Answer from the drawing. Dimensions are ordinates in mm from the lowest x, y and z of the part. Round coordinates to 2 decimals unless told otherwise and drop trailing zeros. Order: outer loops, then holes, each group sorted by start corner. A loop starts at its lowest first (then second) coordinate and runs counter-clockwise, first axis right, second up. Notation, with made-up numbers: (-22.5, 61) -> (10.5, 61) arc R6 cw to (10.5, 65) -> close; hole circle Ø5 at (-20.75, 27). An arc over 180 degrees is marked (long way). Use a Markdown table: item, result. Add a question column.
1. Section A-A, the plane x = 41 is taken. Give the vertices of the cut face in (y, z), then the cut area to 3 significant figures.
2. Section B-B, the plane z = 41 is taken. Give the vertices of the cut face in (x, y).
3. Section C-C, the plane y = 37 is taken. Give the vertices of the cut face in (x, z), then the cut area to 3 significant figures.
4. The mould has two halves that part along X. Classify the marked faces 1 and 2: +X half, -X half, draft (parallel to the pull), parting line (faces both ways), or undercut.
5. Consider L1, parallel to Z at x = 41, y = 47.5; L2, parallel to X at y = 42, z = 40; L3, parallel to Z at x = 45, y = 32.5. Determine where each line is inside the solid, lowest interval first. Write a range as [from, to].
6. Section D-D, the plane y = 20.5 is taken. Give the vertices of the cut face in (x, z).
7. Given pin 1 (2 mm diameter, centred on y = 12.5, z = 10.5, fed in from +X); pin 2 (1.1 mm diameter, centred on x = 79, y = 43, fed in from +Z); pin 3 (4 mm diameter, centred on x = 35, y = 57.5, fed in from +Z), each flat-ended and moving along its own axis, determine where each tip first touches the part or whether it passes through.
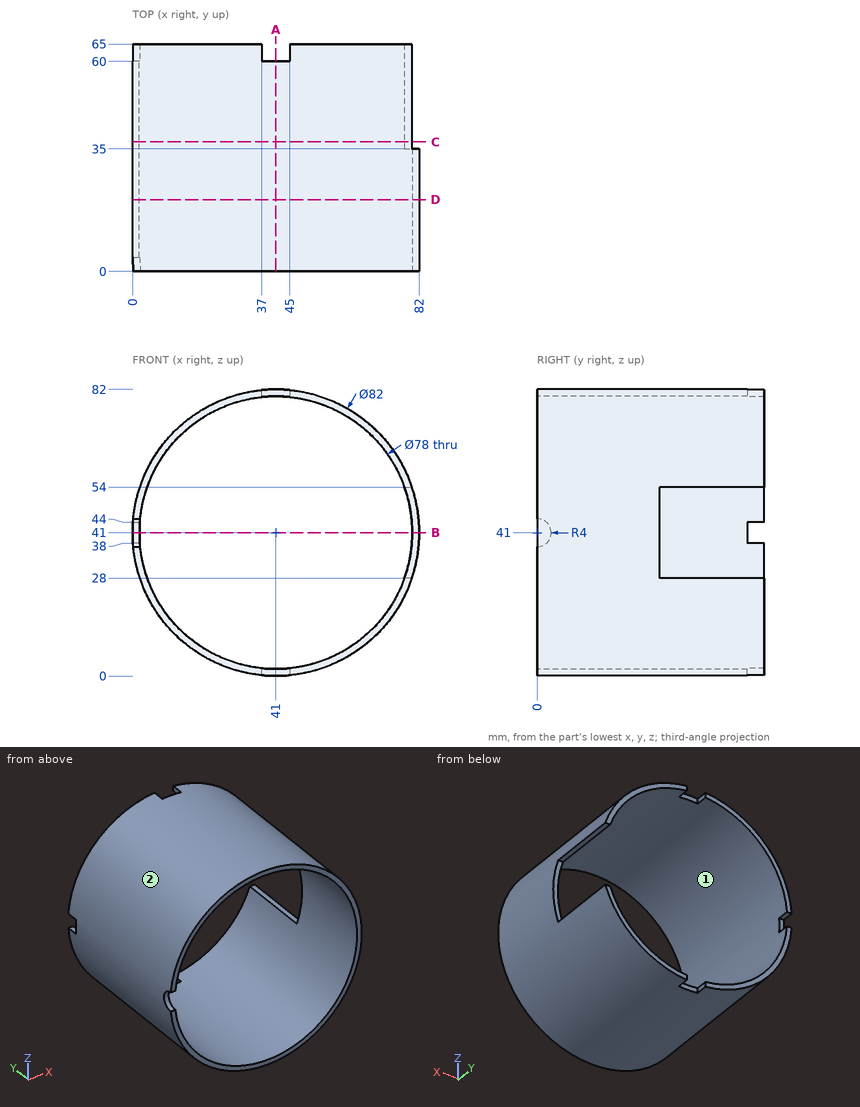
Verdict:
| question | item | result |
|---|---|---|
| 1 | outline | (0, 0) -> (60, 0) -> (60, 2) -> (0, 2) -> close; (0, 80) -> (60, 80) -> (60, 82) -> (0, 82) -> close |
| 1 | area | 240 mm2 |
| 2 | outline | (0, 4) -> (2, 4) -> (2, 60) -> (0, 60) -> close; (80, 0) -> (82, 0) -> (82, 35) -> (80, 35) -> close |
| 3 | outline | (77.77, 28) arc R39 cw (long way) to (77.77, 54) -> (79.88, 54) arc R41 ccw (long way) to (79.88, 28) -> close |
| 3 | area | 450 mm2 |
| 4 | face 1 | undercut |
| 4 | face 2 | parting line |
| 5 | L1 | z = [0, 2], [80, 82] |
| 5 | L2 | x = [0.01, 2.01] |
| 5 | L3 | z = [0.2, 2.21], [79.79, 81.8] |
| 6 | outline | circle Ø82 at (41, 41); hole circle Ø78 at (41, 41) |
| 7 | pin 1 | stops at x = 69.47 |
| 7 | pin 2 | stops at z = 57.69 |
| 7 | pin 3 | stops at z = 81.8 |
